Geometry: final body of the model. Coordinates: model frame, mm. A direction names the side the tool comes from. Round coordinates to 2 decimals unless told otherwise and drop trailing zeros. Loops run counter-clockwise (first coordinate to the right, second up) from the corner with the lowest first, then second, coordinate; pieces in that order, holes last. Notation, with made-up numbers: M 0.25,22.25 L 54.25,22.25 A27 ccw 54.25,45.25 Z; hole C 34,81.5 d8. An arc over 180 degrees is marked long. Write each question's results on one line, items separated by ' | '.
```python
from build123d import *

# Parameters (mm, degrees)
BOSS_EXTRUDE1_DEPTH = 10
SKETCH2_R           = 2.1
SKETCH2_R_2         = 6.5
CUT_EXTRUDE1_DEPTH  = 4
SKETCH3_R           = 6.5
CUT_EXTRUDE2_DEPTH  = 4
SKETCH4_R           = 3
CUT_EXTRUDE3_DEPTH  = 7.0000001
SKETCH7_R           = 1.6
CUT_EXTRUDE6_DEPTH  = 11.0000001
SKETCH8_R           = 2.1
CUT_EXTRUDE7_DEPTH  = 11.0000001


with BuildPart() as part:
    # Sketch1 → Boss-Extrude1 (new body)
    with BuildSketch(Plane.XY):
        with BuildLine():
            Line((10, 0), (11.456439237, 83.439348028))
            ThreePointArc((11.456439237, 83.439348028), (12.5, 88.439348028), (11.456439237, 93.439348028))
            add(Edge.make_bspline(
                [(11.456439237, 93.439348028), (6.1563812, 107.325761573), (5.671965352, 122.191845585)],
                knots=[0, 0, 0, 1, 1, 1], degree=2))
            ThreePointArc((5.671965352, 122.191845585), (0, 127.863810938), (-5.671965352, 122.191845585))
            add(Edge.make_bspline(
                [(-11.456439237, 93.439348028), (-6.1563812, 107.325761573), (-5.671965352, 122.191845585)],
                knots=[0, 0, 0, 1, 1, 1], degree=2))
            ThreePointArc((-11.456439237, 93.439348028), (-12.5, 88.439348028), (-11.456439237, 83.439348028))
            Line((-11.456439237, 83.439348028), (-10, 0))
            Line((-10, 0), (-10, -40))
            Line((-10, -40), (10, -40))
            Line((10, -40), (10, 0))
        make_face()
        Polygon((-7.5, 19.769248097), (-4.375, 14.769248097), (-7.5, 9.769248097), align=None, mode=Mode.SUBTRACT)
        Polygon((-7.5, 44.769248097), (-4.375, 39.769248097), (-7.5, 34.769248097), align=None, mode=Mode.SUBTRACT)
        Polygon((-5, 5.439121078), (0, 13.439121078), (5, 5.439121078), align=None, mode=Mode.SUBTRACT)
        Polygon((0, 16.099375116), (-5, 24.099375116), (5, 24.099375116), align=None, mode=Mode.SUBTRACT)
        Polygon((7.5, 19.769248097), (7.5, 9.769248097), (4.375, 14.769248097), align=None, mode=Mode.SUBTRACT)
        Polygon((-5, 30.439121078), (0, 38.439121078), (5, 30.439121078), align=None, mode=Mode.SUBTRACT)
        Polygon((7.5, 44.769248097), (7.5, 34.769248097), (4.375, 39.769248097), align=None, mode=Mode.SUBTRACT)
        Polygon((-7.5, 69.769248097), (-4.375, 64.769248097), (-7.5, 59.769248097), align=None, mode=Mode.SUBTRACT)
        Polygon((5, 55.439121078), (-5, 55.439121078), (0, 63.439121078), align=None, mode=Mode.SUBTRACT)
        Polygon((0, 66.099375116), (-5, 74.099375116), (5, 74.099375116), align=None, mode=Mode.SUBTRACT)
        Polygon((0, 41.099375116), (-5, 49.099375116), (5, 49.099375116), align=None, mode=Mode.SUBTRACT)
        Polygon((4.375, 64.769248097), (7.5, 69.769248097), (7.5, 59.769248097), align=None, mode=Mode.SUBTRACT)
    extrude(amount=BOSS_EXTRUDE1_DEPTH)

    # Sketch2 → Cut-Extrude1 (cut)
    with BuildSketch(Plane.XY.offset(10)):
        with Locations((0, 122.191845585)):
            Circle(SKETCH2_R)
        with Locations((0, 88.439348028)):
            Circle(SKETCH2_R_2)
    extrude(amount=-CUT_EXTRUDE1_DEPTH, mode=Mode.SUBTRACT)

    # Sketch3 → Cut-Extrude2 (cut)
    with BuildSketch(Plane(origin=(0, 0, 0), x_dir=(-1, 0, 0), z_dir=(0, 0, -1))):
        with Locations((0, 88.439348028)):
            Circle(SKETCH3_R)
    extrude(amount=-CUT_EXTRUDE2_DEPTH, mode=Mode.SUBTRACT)

    # Sketch4 → Cut-Extrude3 (cut, through all)
    with BuildSketch(Plane(origin=(0, 0, 4), x_dir=(-1, 0, 0), z_dir=(0, 0, -1))):
        with Locations((0, 88.439348028)):
            Circle(SKETCH4_R)
    extrude(amount=-CUT_EXTRUDE3_DEPTH, mode=Mode.SUBTRACT)

    # Sketch7 → Cut-Extrude6 (cut, through all)
    with BuildSketch(Plane.XY.offset(10)):
        with Locations((0, -25)):
            Circle(SKETCH7_R)
        with Locations((0, -35)):
            Circle(SKETCH7_R)
    extrude(amount=-CUT_EXTRUDE6_DEPTH, mode=Mode.SUBTRACT)

    # Sketch8 → Cut-Extrude7 (cut, through all)
    with BuildSketch(Plane.XY.offset(10)):
        with Locations((0, 122.191845585)):
            Circle(SKETCH8_R)
    extrude(amount=-CUT_EXTRUDE7_DEPTH, mode=Mode.SUBTRACT)


solid = part.part
```
1. Section B-B (y = 43). Output: boundary loops of the cut face in (x, z).
Answer key:
outline: M -10.75,0 L -7.5,0 L -7.5,10 L -10.75,10 Z; M -6.39,0 L -1.19,0 L -1.19,10 L -6.39,10 Z; M 1.19,0 L 6.39,0 L 6.39,10 L 1.19,10 Z; M 7.5,0 L 10.75,0 L 10.75,10 L 7.5,10 Z
2. Draft query along X for faces 1 (the face through (2.535, 45.155, 4.93)), 2 (the face through (7.5, 40, 5)). Return one class per face: pulls with the +X half, pulls with the -X half, needs draft (parallel to the pull), parting line crosses it, or undercut.
Answer key:
face 1: undercut | face 2: undercut
3. Access query for faces 3 (the face through (-0.846, 94.884, 8.028)), 4 (the face through (0.846, 94.884, 1.972)), 5 (the face through (0, 55.439, 5)). Directions: +Z, -Z, +X, -X, +Y, -Y. A direction counts if a zero-diameter tool reaches every point of the face in a straight line with its end or side. Return the directions, or none.
Answer key:
face 3: +Z | face 4: -Z | face 5: +Z, -Z
4. Ray query, probe 1 along X at (y, z) = (10.5, 2.5); probe 2 along X at (y, z) = (67, 2.75); probe 3 along X at (y, z) = (73.5, 3). Return the intervals inside material, ascending.
Answer key:
probe 1: x = -10.18 to -7.5, -7.04 to -1.84, 1.84 to 7.04, 7.5 to 10.18 | probe 2: x = -11.17 to -7.5, -5.77 to -0.56, 0.56 to 5.77, 7.5 to 11.17 | probe 3: x = -11.28 to -4.63, 4.63 to 11.28
5. Section A-A (y = -35). Output: boundary loops of the cut face in (x, z).
Answer key:
outline: M -10,0 L -1.6,0 L -1.6,10 L -10,10 Z; M 1.6,0 L 10,0 L 10,10 L 1.6,10 Z
6. Pin query (flat end, axial travel): P1, Ø1, axis at y = 11, z = 4, coming from the -X side; P2, Ø6.5, axis at x = 0.5, y = 88, coming from the +Z side; P3, Ø4, axis at x = 1.5, y = 90, coming from the -Z side; P4, Ø3, axis at x = 0, y = -35, coming from the +Z side. Return the tip coordinate at first contact, or that it passes through.
Answer key:
P1: stops at x = -10.2 | P2: stops at z = 6 | P3: stops at z = 4 | P4: passes through
7. Section C-C (z = 2.25). Count the separate pieces of the cut face and the enclosed holes in it, then the cut area to 3 significant figures.
Answer key:
separate pieces: 1 | enclosed holes: 16 | area: 2,830 mm²
